from build123d import *

# Parameters (mm, degrees)
CROQUIS2_R                                           = 1.3
SALIENTE_EXTRUIR1_DEPTH                              = 6.5
SALIENTE_EXTRUIR1_2_DEPTH                            = 6.5
SALIENTE_EXTRUIR1_3_DEPTH                            = 6.5
SALIENTE_EXTRUIR1_4_DEPTH                            = 6.5
CROQUIS3_R                                           = 2.5
SALIENTE_EXTRUIR2_DEPTH                              = 5
CROQUIS4_R                                           = 0.75
CORTAR_EXTRUIR1_DEPTH                                = 5
SALIENTE_EXTRUIR3_DEPTH                              = 4
SALIENTE_EXTRUIR4_DEPTH                              = 45
SALIENTE_EXTRUIR4_DEPTH_BACK                         = 4
REDONDEO1_R                                          = 4
CORTAR_EXTRUIR2_DEPTH                                = 5
CROQUIS8_R                                           = 10.5
CORTAR_EXTRUIR3_DEPTH                                = 5
CROQUIS9_R                                           = 4
SALIENTE_EXTRUIR6_DEPTH                              = 45
REFRENTADO_PARA_TORNILLO_TAP_N_CON_CABEZ_D           = 2.5
REFRENTADO_PARA_TORNILLO_TAP_N_CON_CABEZ_DEPTH       = 10
REFRENTADO_PARA_TORNILLO_TAP_N_CON_CABEZ_CSINK_D     = 4
REFRENTADO_PARA_TORNILLO_TAP_N_CON_CABEZ_CSINK_ANGLE = 90
REFRENTADO_PARA_TORNILLO_TAP_N_CON_CABEZ_TIP         = 0.751075774
REFRENTADO_PARA_TORNILLO_TAP_N_CON_C_2_D             = 4.5
REFRENTADO_PARA_TORNILLO_TAP_N_CON_C_2_DEPTH         = 10
REFRENTADO_PARA_TORNILLO_TAP_N_CON_C_2_CSINK_D       = 8.96
REFRENTADO_PARA_TORNILLO_TAP_N_CON_C_2_CSINK_ANGLE   = 90
REFRENTADO_PARA_TORNILLO_TAP_N_CON_C_2_TIP           = 1.351936393


with BuildPart() as part:
    # Croquis2 → Saliente-Extruir1 (new body)
    with BuildSketch(Plane(origin=(0, 0, 0), x_dir=(1, 0, 0), z_dir=(0, 1, 0))):
        with Locations(Location((3, 3, 0), (0, 0, 90))):
            Circle(CROQUIS2_R)
    extrude(amount=SALIENTE_EXTRUIR1_DEPTH)



with BuildPart() as body_2:
    # Croquis2 → Saliente-Extruir1 2 (new body)
    with BuildSketch(Plane(origin=(0, 0, 0), x_dir=(1, 0, 0), z_dir=(0, 1, 0))):
        with Locations(Location((111.3361, 3, 0), (0, 0, 90))):
            Circle(CROQUIS2_R)
    extrude(amount=SALIENTE_EXTRUIR1_2_DEPTH)


with BuildPart() as body_3:
    # Croquis2 → Saliente-Extruir1 3 (new body)
    with BuildSketch(Plane(origin=(0, 0, 0), x_dir=(1, 0, 0), z_dir=(0, 1, 0))):
        with Locations(Location((109.6374, 43.2299, 0), (0, 0, 90))):
            Circle(CROQUIS2_R)
    extrude(amount=SALIENTE_EXTRUIR1_3_DEPTH)


with BuildPart() as body_4:
    # Croquis2 → Saliente-Extruir1 4 (new body)
    with BuildSketch(Plane(origin=(0, 0, 0), x_dir=(1, 0, 0), z_dir=(0, 1, 0))):
        with Locations(Location((3, 45, 0), (0, 0, 90))):
            Circle(CROQUIS2_R)
    extrude(amount=SALIENTE_EXTRUIR1_4_DEPTH)


with BuildPart() as part_1:
    add(part.part)

    add(body_2.part)  # Saliente-Extruir2 merges body 2

    add(body_3.part)  # Saliente-Extruir2 merges body 3

    add(body_4.part)  # Saliente-Extruir2 merges body 4
    # Croquis3 → Saliente-Extruir2 (add)
    with BuildSketch(Plane(origin=(0, 0, 0), x_dir=(1, 0, 0), z_dir=(0, 1, 0))):
        with Locations(Location((3, 45, 0), (0, 0, 270))):
            Circle(CROQUIS3_R)
        with Locations(Location((3, 3, 0), (0, 0, 270))):
            Circle(CROQUIS3_R)
        with Locations(Location((111.3361, 3, 0), (0, 0, 270))):
            Circle(CROQUIS3_R)
        with Locations(Location((109.6374, 43.2299, 0), (0, 0, 270))):
            Circle(CROQUIS3_R)
    extrude(amount=SALIENTE_EXTRUIR2_DEPTH)

    # Croquis4 → Cortar-Extruir1 (cut)
    with BuildSketch(Plane(origin=(0, 6.5, 0), x_dir=(1, 0, 0), z_dir=(0, 1, 0))):
        with Locations(Location((3, 45, 0), (0, 0, 270))):
            Circle(CROQUIS4_R)
        with Locations(Location((3, 3, 0), (0, 0, 270))):
            Circle(CROQUIS4_R)
        with Locations(Location((111.3361, 3, 0), (0, 0, 270))):
            Circle(CROQUIS4_R)
        with Locations(Location((109.6374, 43.2299, 0), (0, 0, 270))):
            Circle(CROQUIS4_R)
    extrude(amount=-CORTAR_EXTRUIR1_DEPTH, mode=Mode.SUBTRACT)

    # Croquis5 → Saliente-Extruir3 (add)
    with BuildSketch(Plane(origin=(0, 0, 0), x_dir=(1, 0, 0), z_dir=(0, 1, 0))):
        Polygon((124.3681, 63.2781), (-64.9319, 63.2781), (-64.9319, 25.0181), (-14.9319, 25.0181), (-14.9319, -14.9819), (124.3681, -14.9819), align=None)
    extrude(amount=-SALIENTE_EXTRUIR3_DEPTH)

    # Croquis6 → Saliente-Extruir4 (add, two sides: drawn at the far end of the back side and taken through both)
    with BuildSketch(Plane(origin=(0, 0, 0), x_dir=(1, 0, 0), z_dir=(0, 1, 0)).offset(-SALIENTE_EXTRUIR4_DEPTH_BACK)):
        Polygon((-68.9319, 21.0181), (-68.9319, 17.0181), (-18.9319, 17.0181), (-18.9319, -18.9819), (128.3681, -18.9819), (128.3681, 67.2781), (-68.9319, 67.2781), align=None)
        Polygon((-14.9319, -14.9819), (124.3681, -14.9819), (124.3681, 63.2781), (-64.9319, 63.2781), (-64.9319, 25.0181), (-14.9319, 25.0181), align=None, mode=Mode.SUBTRACT)
    extrude(amount=SALIENTE_EXTRUIR4_DEPTH + SALIENTE_EXTRUIR4_DEPTH_BACK)

    # Redondeo1
    redondeo1_edges = [part_1.edges().sort_by_distance(p)[0] for p in [
        (-14.9319, 22.5, -25.0181),
        (-64.9319, 22.5, -25.0181),
        (-64.9319, 22.5, -63.2781),
        (124.3681, 22.5, -63.2781),
        (124.3681, 22.5, 14.9819),
        (-14.9319, 22.5, 14.9819),
        (-18.9319, 20.5, -17.0181),
        (-43.9319, -4, -17.0181),
        (-68.9319, 20.5, -17.0181),
        (-68.9319, -4, -42.1481),
        (-68.9319, 20.5, -67.2781),
        (29.7181, -4, -67.2781),
        (128.3681, 20.5, -67.2781),
        (128.3681, -4, -24.1481),
        (128.3681, 20.5, 18.9819),
        (54.7181, -4, 18.9819),
        (-18.9319, 20.5, 18.9819),
        (-18.9319, -4, 0.9819),
    ]]
    fillet(redondeo1_edges, radius=REDONDEO1_R)

    # Croquis7 → Cortar-Extruir2 (cut)
    with BuildSketch(Plane.XY.offset(-17.0181)):
        Polygon((-58.076981595, 22.5), (-51.004440798, 10.25), (-36.859359202, 10.25), (-29.786818405, 22.5), (-36.859359202, 34.75), (-51.004440798, 34.75), align=None)
    extrude(amount=-CORTAR_EXTRUIR2_DEPTH, mode=Mode.SUBTRACT)

    # Croquis8 → Cortar-Extruir3 (cut)
    with BuildSketch(Plane.XY.offset(-22.0181)):
        with Locations((-43.9319, 22.5)):
            Circle(CROQUIS8_R)
    extrude(amount=-CORTAR_EXTRUIR3_DEPTH, mode=Mode.SUBTRACT)

    # Croquis9 → Saliente-Extruir6 (add)
    with BuildSketch(Plane(origin=(0, 45, 0), x_dir=(1, 0, 0), z_dir=(0, 1, 0))):
        with Locations((-64.9319, 63.2781)):
            Circle(CROQUIS9_R)
        with Locations((124.3681, 63.2781)):
            Circle(CROQUIS9_R)
        with Locations((124.3681, -14.9819)):
            Circle(CROQUIS9_R)
        with Locations((-64.9319, 21.0181)):
            Circle(CROQUIS9_R)
        with Locations((-18.9319, 21.0181)):
            Circle(CROQUIS9_R)
        with Locations((-14.9319, -14.9819)):
            Circle(CROQUIS9_R)
        with Locations((29.7181, 63.2781)):
            Circle(CROQUIS9_R)
    extrude(amount=-SALIENTE_EXTRUIR6_DEPTH)

    # Refrentado para tornillo tap_n con cabez
    with Locations(Plane(origin=(0, 45, 0), x_dir=(1, 0, 0), z_dir=(0, 1, 0))):
        with Locations((-64.9319, 21.0181), (-64.9319, 63.2781), (29.7181, 63.2781), (124.3681, 63.2781), (124.3681, -14.9819), (-14.9319, -14.9819), (-18.9319, 21.0181)):
            CounterSinkHole(REFRENTADO_PARA_TORNILLO_TAP_N_CON_CABEZ_D / 2, REFRENTADO_PARA_TORNILLO_TAP_N_CON_CABEZ_CSINK_D / 2, depth=REFRENTADO_PARA_TORNILLO_TAP_N_CON_CABEZ_DEPTH, counter_sink_angle=REFRENTADO_PARA_TORNILLO_TAP_N_CON_CABEZ_CSINK_ANGLE)
            with Locations((0, 0, -(REFRENTADO_PARA_TORNILLO_TAP_N_CON_CABEZ_DEPTH + REFRENTADO_PARA_TORNILLO_TAP_N_CON_CABEZ_TIP / 2))):  # 118° drill point
                Cone(0, REFRENTADO_PARA_TORNILLO_TAP_N_CON_CABEZ_D / 2, REFRENTADO_PARA_TORNILLO_TAP_N_CON_CABEZ_TIP, mode=Mode.SUBTRACT)

    # Refrentado para tornillo tap_n con c 2
    with Locations(Plane(origin=(0, 0, 0), x_dir=(1, 0, 0), z_dir=(0, 1, 0))):
        with Locations((14.6331, 52.5081), (94.8031, 52.5081), (94.8031, -4.2119), (14.6331, -4.2119)):
            CounterSinkHole(REFRENTADO_PARA_TORNILLO_TAP_N_CON_C_2_D / 2, REFRENTADO_PARA_TORNILLO_TAP_N_CON_C_2_CSINK_D / 2, depth=REFRENTADO_PARA_TORNILLO_TAP_N_CON_C_2_DEPTH, counter_sink_angle=REFRENTADO_PARA_TORNILLO_TAP_N_CON_C_2_CSINK_ANGLE)
            with Locations((0, 0, -(REFRENTADO_PARA_TORNILLO_TAP_N_CON_C_2_DEPTH + REFRENTADO_PARA_TORNILLO_TAP_N_CON_C_2_TIP / 2))):  # 118° drill point
                Cone(0, REFRENTADO_PARA_TORNILLO_TAP_N_CON_C_2_D / 2, REFRENTADO_PARA_TORNILLO_TAP_N_CON_C_2_TIP, mode=Mode.SUBTRACT)


solid = part_1.part
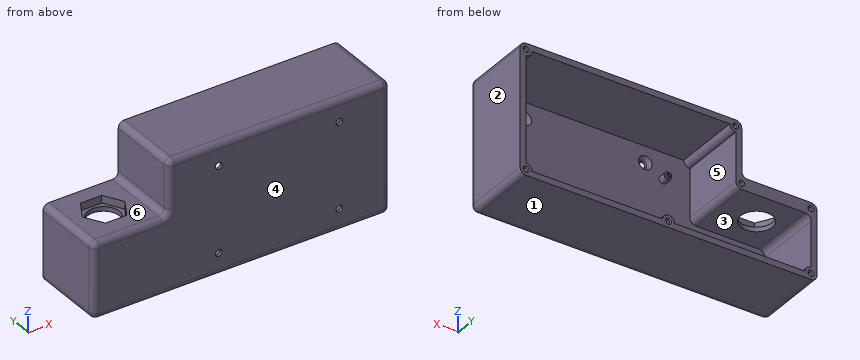
Verification items for the finished model (mm, model axes). Face numbers are marked on the shaded views. A direction names the side the tool comes from. Give positions to 0.01 mm unless a question says otherwise; leave off trailing zeros. Order: outer loops, then holes, each group sorted by start corner. A loop starts at its lowest first (then second) coordinate and runs counter-clockwise, first axis right, second up. Notation, with made-up numbers: M 27,78.5 L 54,78.5 A20 cw 54,102.5 Z; hole C 26.5,83 d5. An arc over 180 degrees is marked long. Use one line per item in the form item = value. Start each with the question number.
Q1. Access from +Z, -Z, +X, -X, +Y, -Y to the whole of each face (thin tool, end or side, straight path). Record for the marked faces 4, 5 and 6.
Q2. Scan lines: line 1 along Z through (x, y) = (102, 12.5); line 2 along X through (y, z) = (-1, 3); line 3 along Y through (x, z) = (-44.5, -50). Record each from-to range of solid material in increasing order. Write a range as [from, to].
Q3. Mould release check, pull along X, two halves, no side actions. Record for the marked faces 1, 2 and 3: +X half, -X half, draft (parallel to the pull), parting line (faces both ways), or undercut.
Q4. Go/stop test with flat-tipped pins: pin 1 Ø10 at (x, z) = (48.5, -35) entering from +Y; pin 2 Ø8 at (y, z) = (16.5, -2.5) entering from -X; pin 3 Ø1.2 at (x, z) = (3, -3) entering from +Y; pin 4 Ø2.5 at (x, z) = (94.8, -52.51) entering from -Y. Record where each tip stops, or that it passes through.
Q5. Section check A-A (z = -34). Enter the section's corners in (x, y).
Q6. Section check B-B (x = 65). Enter the section's corners in (y, z), then the cut area to 3 significant figures.
Evaluation:
q1.face_4 = +Z, -Z, +X, -X, -Y
q1.face_5 = +Y
q1.face_6 = +Z, -X, +Y, -Y
q2.line_1 = [-67.28, -63.28], [14.98, 18.98]
q2.line_2 = [-18.8, 11.37], [17.9, 91.54], [98.07, 128.24]
q2.line_3 = [-4, 0]
q3.face_1 = draft
q3.face_2 = +X half
q3.face_3 = undercut
q4.pin_1 = 0
q4.pin_2 = -18.93
q4.pin_3 = 1.5
q4.pin_4 = through
q5.outline = M -68.93,0 A4 ccw -64.93,-4 L 124.37,-4 A4 ccw 128.37,0 L 128.37,45 L 124.37,45 L 124.37,0 L -64.93,0 L -64.93,45 L -68.93,45 Z
q6.outline = M -4,-63.28 A4 ccw 0,-67.28 L 45,-67.28 L 45,-63.28 L 0,-63.28 L 0,14.98 L 45,14.98 L 45,18.98 L 0,18.98 A4 ccw -4,14.98 Z
q6.area = 698 mm2
